Autodesk Inventor part; units mm, degrees
ref_plane "YZ Plane" through (0, 0, 0) normal (1, 0, 0) x (0, 1, 0)
ref_plane "XZ Plane" through (0, 0, 0) normal (0, 1, 0) x (-1, 0, 0)
ref_plane "XY Plane" through (0, 0, 0) normal (0, 0, 1) x (1, 0, 0)
sketch "草图1" plane through (0, 0, 0) normal (0, 1, 0) x (-1, 0, 0)
  line L0 (0, 0) -> (65, 0)
  line L1 (65, 0) -> (65, -65)
  line L2 (65, -65) -> (0, -65)
  line L3 (0, -65) -> (0, 0)
  dimension "d0" = 65
  dimension "d1" = 65
extrude "拉伸1" add sketch "草图1" along normal blind 10
chamfer "倒角1" distance 65 angle 7 1 edges at (-32.5, 10, 0) measured on face at (-21.6667, 10, -43.3333)
sketch "草图2" plane through (0, 0, 0) normal (0, -1, 0) x (1, 0, 0)
  line L0 (-65, 0) -> (0, 0)
  line L1 (-32.5, 0) -> (-32.5, -65)
  line L2 (0, -65) -> (-65, -65)
  circle A0 centre (-32.5, -32.5) radius 1.95
  dimension "d7" = 3.9
extrude "拉伸2" cut sketch "草图2" against normal blind 4
sketch "草图4" plane through (0, 0, 0) normal (0, -1, 0) x (1, 0, 0)
  line L0 (0, 0) -> (0, -65)
  line L1 (0, -65) -> (-65, -65)
  line L2 (0, 0) -> (-5, 0)
  line L3 (-5, 0) -> (-5, -65)
  line L4 (-5, -65) -> (0, -65)
  line L5 (0, -65) -> (0, 0)
  dimension "d13" = 5
extrude "拉伸4" add sketch "草图4" along normal blind 60
sketch "草图5" plane through (-65, 10, -65) normal (0, 0.9925, 0.1219) x (1, 0, 0)
  line L0 (0, 0) -> (3, 0)
  line L1 (3, 0) -> (3, -35.2725)
  line L2 (3, -35.2725) -> (0, -35.2725)
  line L3 (0, -35.2725) -> (0, 0)
  line L4 (0, -65.4881) -> (65, -65.4881)
  line L5 (0, 0) -> (3, 0)
  line L6 (3, 0) -> (3, -65.4881)
  line L7 (3, -65.4881) -> (0, -65.4881)
  line L8 (0, -65.4881) -> (0, 0)
  point P0 (65, -65.7342)
  point P1 (0, -35.2725)
  point P2 (0, -65.4881)
  point P3 (3, -35.2725)
  dimension "d17" = 3
extrude "拉伸5" add sketch "草图5" along normal blind 65
sketch "草图6" plane through (0, 0, 0) normal (0, -1, 0) x (1, 0, 0)
  line L0 (0, -65) -> (-62, -65)
  line L1 (-65, 0) -> (-4.9882, 0)
  line L2 (-4.9882, 0) -> (-4.9882, -65)
  line L3 (-4.9882, -65) -> (-65, -65)
  line L4 (-65, -65) -> (-65, 0)
  point P0 (0, 0)
extrude "拉伸6" add sketch "草图6" along normal blind 10
sketch "草图8" plane through (0, -10, 0) normal (0, -1, 0) x (1, 0, 0)
  circle A0 centre (-32.5, -32.5) radius 1.95
  circle A1 centre (-32.5, -32.5) radius 2
  point P0 (0, 0)
  dimension "d25" = 4
extrude "拉伸8" cut sketch "草图8" against normal blind 13 contours A0 | A1
equation "\"折弯半径\" = 厚度"
equation "\"折弯释压宽度\" = 厚度"
equation "\"折弯释压深度\" = 0.5 * 厚度"
equation "\"拐角释压尺寸\" = 4 * 厚度"
equation "\"最小余量\" = 2 * 厚度"
equation "\"过渡半径\" = 折弯半径"
equation "\"Jacobi半径尺寸\" = 折弯半径"
equation "\"间隙大小\" = 厚度"
properties part number "_3D 打印"
Read the model definition and answer for the solid it produces. Units are mm, in the model's axes. A direction names the side the tool comes from. Round coordinates to 2 decimals unless told otherwise and drop trailing zeros. Write each loop counter-clockwise with the first axis right and the second up, starting at its lowest first coordinate (ties: lowest second). Pieces come first, ordered by that corner, then holes.
1. The part is cut by section C-C, the plane y = -42.5. Determine the outline of the cut face in (x, z).
2. Which of the six approach directions +Z, -Z, +X, -X, +Y, -Y give full straight-line access (tool end or side, diameter ignored) to faces 1 (the face through (-35, -10, -32)), 2 (the face through (-63.521, 33.825, 3.905)), 3 (the face through (-33, 4, -32))?
3. The part is cut by section D-D, the plane z = -19.5. Determine the outline of the cut face in (x, y).
4. Given pin 1 Ø2 at (x, z) = (-32, -32.5) entering from -Y; pin 2 Ø2 at (x, y) = (-7.5, -10) entering from +Z; pin 3 Ø10 at (x, z) = (-24, -42.5) entering from +Y; pin 4 Ø10 at (y, z) = (-41, -16.5) entering from +X, each flat-ended and moving along its own axis, determine where each tip first touches the part or whether it passes through.
5. The part is cut by section B-B, the plane z = -32.5. Determine the outline of the cut face in (x, y).
6. Straight lines are drawn through the part: L1, parallel to Z at x = -32.5, y = -3.5; L2, parallel to X at y = -4, z = -32. For each, find the intervals that lie inside material, in ascending order.
7. Determine the mould class of faces 4 (the face through (-25, -9, -65)), 5 (the face through (-30.566, 5.954, -32.045)), 6 (the face through (-5, -35, -32)), 7 (the face through (-32.754, 3.493, -30.567)) for opening direction Z: pulls with the +Z half, pulls with the -Z half, needs draft (parallel to the pull), parting line crosses it, or undercut.
Values:
1. outline: (-5, -65) - (0, -65) - (0, 0) - (-5, 0) - close
2. face 1: +Z, -Z, -X, -Y
2. face 2: +Z, +X, -X, -Y
2. face 3: -Y
3. outline: (-65, -10) - (-5, -10) - (-5, -60) - (0, -60) - (0, 4.41) - (-62, 4.41) - (-62, 69.9) - (-65, 69.9) - close
4. pin 1: stops at y = 4
4. pin 2: stops at z = 0
4. pin 3: stops at y = 7.85
4. pin 4: stops at x = 0
5. outline: (-65, -10) - (-34.5, -10) - (-34.5, 3) - (-34.45, 3) - (-34.45, 4) - (-30.55, 4) - (-30.55, 3) - (-30.5, 3) - (-30.5, -10) - (-5, -10) - (-5, -60) - (0, -60) - (0, 6.01) - (-62, 6.01) - (-62, 71.5) - (-65, 71.5) - close
6. L1: z = -65 to -34.5, -30.5 to 0
6. L2: x = -65 to -34.44, -30.56 to 0
7. face 4: pulls with the -Z half
7. face 5: pulls with the +Z half
7. face 6: needs draft
7. face 7: undercut
